from build123d import *

# Parameters (mm, degrees)
BOSS_EXTRUDE1_DEPTH     = 7
CUT_EXTRUDE1_DEPTH      = 12.66243971
CUT_EXTRUDE1_DEPTH_BACK = 12.66243971
SKETCH5_R               = 1.4


with BuildPart() as part:
    # Sketch2 → Revolve1 (revolve)
    with BuildSketch(Plane(origin=(0, 0, 0), x_dir=(0, 0, -1), z_dir=(1, 0, 0)), mode=Mode.PRIVATE) as revolve1_sk:
        Polygon((0, 1.55), (0, 6.05), (1, 6.05), (1, 3.55), (6, 3.55), (6, 6.05), (7, 6.05), (7, 1.55), align=None)
    revolve(revolve1_sk.sketch.rotate(Axis((0, 0, 2.14137931), (0, 0, -1)), 90), axis=Axis((0, 0, 2.14137931), (0, 0, -1)))

    # Sketch4 → Boss-Extrude1 (add)
    with BuildSketch(Plane.XY):
        with BuildLine():
            ThreePointArc((1.140175425, 1.05), (0, 1.55), (-1.140175425, 1.05))
            Line((-1.140175425, 1.05), (1.140175425, 1.05))
        make_face()
    extrude(amount=-BOSS_EXTRUDE1_DEPTH)

    # Sketch5 → Cut-Extrude1 (cut, two sides: drawn at the far end of the back side and taken through both)
    with BuildSketch(Plane.XZ.offset(-1.05).offset(-CUT_EXTRUDE1_DEPTH_BACK)):
        with Locations(Location((0, -3.5, 0), (0, 0, 270))):
            Circle(SKETCH5_R)
    extrude(amount=CUT_EXTRUDE1_DEPTH + CUT_EXTRUDE1_DEPTH_BACK, mode=Mode.SUBTRACT)


solid = part.part
Here's how the part is built. I have some questions about the finished solid (model axes, mm). A direction names the side the tool comes from. Coordinates: 2 decimals unless noted, no trailing zeros. Loops run counter-clockwise (first coordinate to the right, second up) from the corner with the lowest first, then second, coordinate; pieces in that order, holes last.
1. I need wall thicknesses on L1, parallel to Z at x = 0, y = 2.45; L2, parallel to Z at x = 3, y = 2; L3, parallel to Y at x = -1.25, z = -5. Which ranges of each line are inside material? Lowest first, please.
2. Imagine slicing it at C-C, the plane z = -3.5. Please give me the cut outline in (x, y), and give its area (3 significant figures).
3. Imagine slicing it at A-A, the plane y = 0. Please give me the cut outline in (x, z), and give its area (3 significant figures).
4. If we mould it in two halves opening along Z, with no side actions, what happens to faces 1 (the flat face through (0.1, 1.3, 0)), 2 (the flat face through (3, 3, -1)), 3 (the flat face through (0, 1.05, -6))? For each: pulls with the +Z half, pulls with the -Z half, needs draft (parallel to the pull), parting line crosses it, or undercut.
5. Imagine slicing it at B-B, the plane x = 0. Please give me the cut outline in (y, z).
6. For faces 4 (the flat face through (-3, 3, -6)), 5 (the flat face through (0, 1.05, -1)), 6 (the cylindrical face through (0.06, 2.13, -2.1)), which set-ups out of +Z, -Z, +X, -X, +Y, -Y let a thin tool reach every point of the face, with its end or its side?
7. Imagine slicing it at D-D, the plane x = -5. Please give me the cut outline in (y, z).
8. For P1, Ø4, axis at x = -4, z = -6, coming from the -Y side; P2, Ø4, axis at y = -1.5, z = -4.5, coming from the +X side; P3, Ø3, axis at y = -4, z = -3.5, coming from the -X side, each with a flat end and sliding along its axis, tell me the tip position at first contact or that it passes through.
Taken from the geometry:
1. L1: z = -7 to -4.9, -2.1 to 0
1. L2: z = -7 to -6, -1 to 0
1. L3: y = -3.32 to -0.92, 0.92 to 3.32
2. outline: (-1.4, -3.26) - (-1.4, -0.67) arc R1.55 cw to (-1.4, 0.67) - (-1.4, 3.26) arc R3.55 ccw to start; (1.4, -3.26) arc R3.55 ccw to (1.4, 3.26) - (1.4, 0.67) arc R1.55 cw to (1.4, -0.67) - close
2. area: 20.0 mm2
3. outline: (-6.05, -7) - (-1.55, -7) - (-1.55, 0) - (-6.05, 0) - (-6.05, -1) - (-3.55, -1) - (-3.55, -6) - (-6.05, -6) - close; (1.55, -7) - (6.05, -7) - (6.05, -6) - (3.55, -6) - (3.55, -1) - (6.05, -1) - (6.05, 0) - (1.55, 0) - close
3. area: 38.0 mm2
4. face 1: pulls with the +Z half
4. face 2: undercut
4. face 3: needs draft
5. outline: (-6.05, -7) - (-1.55, -7) - (-1.55, -4.9) - (-3.55, -4.9) - (-3.55, -6) - (-6.05, -6) - close; (-6.05, -1) - (-3.55, -1) - (-3.55, -2.1) - (-1.55, -2.1) - (-1.55, 0) - (-6.05, 0) - close; (1.05, -7) - (6.05, -7) - (6.05, -6) - (3.55, -6) - (3.55, -4.9) - (1.05, -4.9) - close; (1.05, -2.1) - (3.55, -2.1) - (3.55, -1) - (6.05, -1) - (6.05, 0) - (1.05, 0) - close
6. face 4: none
6. face 5: +Z, -Z
6. face 6: +Y, -Y
7. outline: (-3.41, -7) - (3.41, -7) - (3.41, -6) - (-3.41, -6) - close; (-3.41, -1) - (3.41, -1) - (3.41, 0) - (-3.41, 0) - close
8. P1: stops at y = -5.71
8. P2: stops at x = 6.05
8. P3: stops at x = -2.52
